from build123d import *

# Parameters (mm, degrees)
SKETCH2_W           = 20
SKETCH2_H           = 15
BOSS_EXTRUDE1_DEPTH = 50
CUT_EXTRUDE2_DEPTH  = 20


with BuildPart() as part:
    # Sketch2 → Boss-Extrude1 (new body)
    with BuildSketch(Plane.XY):
        Rectangle(SKETCH2_W, SKETCH2_H)
    extrude(amount=BOSS_EXTRUDE1_DEPTH)

    # Sketch4 → Cut-Extrude2 (cut)
    with BuildSketch(Plane.XY.offset(50)):
        Polygon((-7.5, -2.5), (7.5, -2.5), (7.5, 1.75), (6.65, 1.75), (6.65, 3.25), (7.5, 3.25), (7.5, 7.5), (-7.5, 7.5), (-7.5, 3.25), (-6.65, 3.25), (-6.65, 1.75), (-7.5, 1.75), align=None)
    cut_extrude2 = extrude(amount=-CUT_EXTRUDE2_DEPTH, mode=Mode.SUBTRACT)

    # Mirror1: Cut-Extrude2 across plane
    add(cut_extrude2.mirror(Plane.XY.offset(25)), mode=Mode.SUBTRACT)


solid = part.part
Build history of the part. All positions in model axes, mm. A direction names the side the tool comes from. Coordinates: 2 decimals unless noted, no trailing zeros. Write each loop counter-clockwise with the first axis right and the second up, starting at its lowest first coordinate (ties: lowest second). Pieces come first, ordered by that corner, then holes.
(1) Drill centre lines: line 1 (X direction, y = 0.25, z = 38.5); line 2 (Y direction, x = 7.25, z = 46); line 3 (Y direction, x = 3.75, z = 15.5). Where is each one in solid material? Low to high.
(2) Cut at B-B on x = 6. List the corners of the cut face in (y, z).
(3) 3-axis set-ups, long thin cutter, end or side, ignore diameter. For faces 4 (the flat face through (7, 3.25, 10)), 5 (the flat face through (10, 0, 25)), 6 (the flat face through (7.5, 0, 10)), 7 (the flat face through (7, 1.75, 40)), 8 (the flat face through (-7, 3.25, 40)): which of +Z, -Z, +X, -X, +Y, -Y reach the whole face in a straight line?
(4) Pin check, flat tips, straight feed: pin 1 Ø3 at (x, y) = (0.5, 3.5) entering from +Z; pin 2 Ø1.5 at (x, y) = (-0.5, 1.5) entering from -Z; pin 3 Ø12 at (x, z) = (2, 37) entering from +Y; pin 4 Ø0.9 at (x, z) = (7, 36.5) entering from +Y. Stop position of each tip, or through.
(5) Cut at A-A on z = 46. List the corners of the cut face in (x, y).
(6) Cut at C-C on y = 6.25. List the corners of the cut face in (x, z), and give its area (3 significant figures).
(7) Mould opens along X. For faces 1 (the flat face through (0, -7.5, 25)), 2 (the flat face through (7.5, 5, 40)), 3 (the flat face through (-10, 0, 25)) say: pulls with the +X half, pulls with the -X half, needs draft (parallel to the pull), parting line crosses it, or undercut.
Working result:
1. line 1: x = -10 to -7.5, 7.5 to 10
1. line 2: y = -7.5 to -2.5, 1.75 to 3.25
1. line 3: y = -7.5 to -2.5
2. outline: (-7.5, 0) - (-2.5, 0) - (-2.5, 20) - (7.5, 20) - (7.5, 30) - (-2.5, 30) - (-2.5, 50) - (-7.5, 50) - close
3. face 4: -Z, +Y
3. face 5: +Z, -Z, +X, +Y, -Y
3. face 6: -Z
3. face 7: +Z
3. face 8: +Z, +Y
4. pin 1: stops at z = 30
4. pin 2: stops at z = 20
4. pin 3: stops at y = 7.5
4. pin 4: stops at y = 3.25
5. outline: (-10, -7.5) - (10, -7.5) - (10, 7.5) - (7.5, 7.5) - (7.5, 3.25) - (6.65, 3.25) - (6.65, 1.75) - (7.5, 1.75) - (7.5, -2.5) - (-7.5, -2.5) - (-7.5, 1.75) - (-6.65, 1.75) - (-6.65, 3.25) - (-7.5, 3.25) - (-7.5, 7.5) - (-10, 7.5) - close
6. outline: (-10, 0) - (-7.5, 0) - (-7.5, 20) - (7.5, 20) - (7.5, 0) - (10, 0) - (10, 50) - (7.5, 50) - (7.5, 30) - (-7.5, 30) - (-7.5, 50) - (-10, 50) - close
6. area: 400 mm2
7. face 1: needs draft
7. face 2: undercut
7. face 3: pulls with the -X half
